from build123d import *

# Parameters (mm, degrees)
F1_DEPTH    = 19.05
F2_T2_ANGLE = 47.80727079
F4_DEPTH    = 3.175


# Not quite as in the source:
# - a fillet or chamfer that OpenCascade refuses, or shapes differently, is made with other operations: its cross-section is extruded or revolved along the edge and cut away or added


with BuildPart() as f1:
    # F0 (on Front) → F1 (new body)
    with BuildSketch(Plane.XZ):
        with BuildLine():
            Line((-379.386894745, -118.26875), (379.4125, -118.26875))
            Line((379.4125, -118.26875), (379.4125, -113.50625))
            Line((379.4125, -113.50625), (393.7, -113.50625))
            Line((393.7, -113.50625), (393.7, 124.61875))
            ThreePointArc((393.7, 124.61875), (-0.5889314831, 196.0563533265), (-393.674394745, 118.26875))
            Line((-393.674394745, 118.26875), (-393.674394745, -113.50625))
            Line((-393.674394745, -113.50625), (-379.386894745, -113.50625))
            Line((-379.386894745, -113.50625), (-379.386894745, -118.26875))
        make_face()
        with BuildLine():
            ThreePointArc((-393.674394745, 118.26875), (-0.5889314831, 196.0563533265), (393.7, 124.61875))
            Line((393.7, 124.61875), (393.7, 138.90625))
            ThreePointArc((393.7, 138.90625), (-0.7824585401, 208.7544433839), (-393.7768174305, 130.96875))
            Line((-393.7768174305, 130.96875), (-393.674394745, 118.26875))
        make_face()
    extrude(amount=F1_DEPTH)

    # F2: chamfer of 19.558 x 11.43 on 1 edges, made by hand

    # F2_s1 → F2_t2 (revolve, cut)
    with BuildSketch(Plane(origin=(327.911656241, 0, -141.3984070605), x_dir=(0, 1, 0), z_dir=(0.9182658757, 0, -0.3959643691))):
        Polygon((0.508, 284.621375818), (-19.05, 273.191375818), (-19.05, 284.621375818), align=None)
    revolve(axis=Axis((10.1741912427, -19.05, -878.2512511865), (0, -1, 0)), revolution_arc=F2_T2_ANGLE, mode=Mode.SUBTRACT)

    # F3 (on face) → F4 (join)
    with BuildSketch(Plane.XZ.offset(19.05)):
        Polygon((71.1841804533, -118.26875), (178.9472539061, -118.26875), (218.205169263, -79.0108346431), (164.3236325366, -25.1292979167), (110.4420958102, -79.0108346431), align=None)
        Polygon((218.205169263, -79.0108346431), (178.9472539061, -118.26875), (257.4630846199, -118.26875), align=None)
        Polygon((393.7, -113.50625), (393.7, -38.9795184745), (379.8497794422, -25.1292979167), (325.9682427158, -79.0108346431), (286.710327359, -118.26875), (379.4125, -118.26875), (379.4125, -113.50625), align=None)
        Polygon((379.8497794422, -25.1292979167), (393.7, -38.9795184745), (393.7, -11.279077359), align=None)
        Polygon((218.205169263, -79.0108346431), (257.4630846199, -118.26875), (286.710327359, -118.26875), (325.9682427158, -79.0108346431), (272.0867059894, -25.1292979167), (218.205169263, 28.7522388097), (164.3236325366, -25.1292979167), align=None)
        Polygon((41.9369377142, -118.26875), (71.1841804533, -118.26875), (110.4420958102, -79.0108346431), (56.5605590837, -25.1292979167), (2.6790223573, 28.7522388097), (-51.2025143691, -25.1292979167), (2.6790223573, -79.0108346431), align=None)
        Polygon((-36.5788929995, -118.26875), (41.9369377142, -118.26875), (2.6790223573, -79.0108346431), align=None)
        Polygon((-144.3419664524, -118.26875), (-36.5788929995, -118.26875), (2.6790223573, -79.0108346431), (-51.2025143691, -25.1292979167), (-105.0840510955, -79.0108346431), align=None)
        Polygon((325.9682427158, -79.0108346431), (379.8497794422, -25.1292979167), (393.7, -11.279077359), (393.7, 68.7835549784), (379.8497794422, 82.6337755361), (325.9682427158, 28.7522388097), (272.0867059894, -25.1292979167), align=None)
        Polygon((110.4420958102, -79.0108346431), (164.3236325366, -25.1292979167), (218.205169263, 28.7522388097), (164.3236325366, 82.6337755361), (110.4420958102, 28.7522388097), (56.5605590837, -25.1292979167), align=None)
        Polygon((-173.5892091915, -118.26875), (-144.3419664524, -118.26875), (-105.0840510955, -79.0108346431), (-158.9655878219, -25.1292979167), (-212.8471245483, 28.7522388097), (-266.7286612747, -25.1292979167), (-212.8471245483, -79.0108346431), align=None)
        Polygon((379.8497794422, 82.6337755361), (393.7, 68.7835549784), (393.7, 96.4839960939), align=None)
        Polygon((218.205169263, 28.7522388097), (272.0867059894, -25.1292979167), (325.9682427158, 28.7522388097), (272.0867059894, 82.6337755361), (218.205169263, 136.5153122625), (164.3236325366, 82.6337755361), align=None)
        Polygon((2.6790223573, 28.7522388097), (56.5605590837, -25.1292979167), (110.4420958102, 28.7522388097), (56.5605590837, 82.6337755361), (2.6790223573, 136.5153122625), (-51.2025143691, 82.6337755361), align=None)
        Polygon((-105.0840510955, -79.0108346431), (-51.2025143691, -25.1292979167), (2.6790223573, 28.7522388097), (-51.2025143691, 82.6337755361), (-105.0840510955, 28.7522388097), (-158.9655878219, -25.1292979167), align=None)
        Polygon((-252.1050399052, -118.26875), (-173.5892091915, -118.26875), (-212.8471245483, -79.0108346431), align=None)
        Polygon((-359.868113358, -118.26875), (-252.1050399052, -118.26875), (-212.8471245483, -79.0108346431), (-266.7286612747, -25.1292979167), (-320.6101980012, -79.0108346431), align=None)
        with BuildLine():
            Line((325.9682427158, 28.7522388097), (379.8497794422, 82.6337755361))
            Line((379.8497794422, 82.6337755361), (393.7, 96.4839960939))
            Line((393.7, 96.4839960939), (393.7, 126.6814901711))
            ThreePointArc((393.7, 126.6814901711), (365.104665334, 137.1335129285), (336.2249713921, 146.7720409389))
            Line((336.2249713921, 146.7720409388), (325.9682427158, 136.5153122625))
            Line((325.9682427158, 136.5153122625), (272.0867059894, 82.6337755361))
            Line((272.0867059894, 82.6337755361), (325.9682427158, 28.7522388097))
        make_face()
        with BuildLine():
            Line((110.4420958102, 28.7522388097), (164.3236325366, 82.6337755361))
            Line((164.3236325366, 82.6337755361), (218.205169263, 136.5153122625))
            Line((218.205169263, 136.5153122625), (169.1544903585, 185.565991167))
            ThreePointArc((169.1544903585, 185.565991167), (164.9380697375, 186.1875692954), (160.7192193307, 186.792435783))
            Line((160.7192193307, 186.792435783), (110.4420958102, 136.5153122625))
            Line((110.4420958102, 136.5153122625), (56.5605590837, 82.6337755361))
            Line((56.5605590837, 82.6337755361), (110.4420958102, 28.7522388097))
        make_face()
        Polygon((-212.8471245483, 28.7522388097), (-158.9655878219, -25.1292979167), (-105.0840510955, 28.7522388097), (-158.9655878219, 82.6337755361), (-212.8471245483, 136.5153122625), (-266.7286612747, 82.6337755361), align=None)
        with BuildLine():
            Line((218.205169263, 136.5153122625), (272.0867059894, 82.6337755361))
            Line((272.0867059894, 82.6337755361), (325.9682427158, 136.5153122625))
            Line((325.9682427158, 136.5153122625), (306.8177631195, 155.6657918589))
            ThreePointArc((306.8177631195, 155.6657918589), (238.4761479453, 172.8719942997), (169.1544903585, 185.565991167))
            Line((169.1544903585, 185.565991167), (218.205169263, 136.5153122625))
        make_face()
        with BuildLine():
            Line((2.6790223573, 136.5153122625), (56.5605590838, 82.6337755361))
            Line((56.5605590837, 82.6337755361), (110.4420958102, 136.5153122625))
            Line((110.4420958102, 136.5153122625), (56.5605590837, 190.3968489889))
            Line((56.5605590837, 190.3968489889), (50.3274681554, 196.6299399173))
            ThreePointArc((50.3274681554, 196.6299399173), (2.3207372282, 197.350991232), (-45.670346508, 195.92901685))
            Line((-45.670346508, 195.92901685), (-51.2025143691, 190.3968489889))
            Line((-51.2025143691, 190.3968489889), (2.6790223573, 136.5153122625))
        make_face()
        Polygon((-105.0840510955, 28.7522388097), (-51.2025143691, 82.6337755361), (2.6790223573, 136.5153122625), (-51.2025143691, 190.3968489889), (-105.0840510955, 136.5153122625), (-158.9655878219, 82.6337755361), align=None)
        Polygon((-266.7286612747, -25.1292979167), (-212.8471245483, 28.7522388097), (-266.7286612747, 82.6337755361), (-320.6101980012, 28.7522388097), (-374.4917347276, -25.1292979167), (-320.6404889111, -78.9805437332), (-320.6101980012, -79.0108346431), align=None)
        Polygon((-379.386894745, -118.26875), (-359.9286951779, -118.26875), (-320.6404889111, -78.9805437332), (-374.4917347276, -25.1292979167), (-393.674394745, -5.9466378993), (-393.674394745, -113.50625), (-379.386894745, -113.50625), align=None)
        with BuildLine():
            Line((325.9682427158, 136.5153122625), (336.2249713921, 146.7720409388))
            ThreePointArc((336.2249713921, 146.7720409389), (321.5531223101, 151.3239145605), (306.8177631195, 155.6657918589))
            Line((306.8177631195, 155.6657918589), (325.9682427158, 136.5153122625))
        make_face()
        with BuildLine():
            Line((56.5605590837, 190.3968489889), (110.4420958102, 136.5153122625))
            Line((110.4420958102, 136.5153122625), (160.7192193307, 186.792435783))
            ThreePointArc((160.7192193307, 186.792435783), (111.6070850178, 192.5863782868), (62.2805468294, 196.1168367345))
            Line((62.2805468293, 196.1168367345), (56.5605590837, 190.3968489889))
        make_face()
        with BuildLine():
            Line((-320.6101980012, 28.7522388097), (-266.7286612747, 82.6337755361))
            Line((-266.7286612747, 82.6337755361), (-212.8471245483, 136.5153122625))
            Line((-212.8471245483, 136.5153122625), (-243.3958660177, 167.0640537319))
            ThreePointArc((-243.3958660177, 167.0640537319), (-275.7499582928, 158.6813605815), (-307.8279930641, 149.2975171996))
            Line((-307.8279930641, 149.2975171996), (-320.6101980012, 136.5153122625))
            Line((-320.6101980012, 136.5153122625), (-374.4917347276, 82.6337755361))
            Line((-374.4917347276, 82.6337755361), (-320.6101980012, 28.7522388097))
        make_face()
        with BuildLine():
            Line((-212.8471245483, 136.5153122625), (-158.9655878219, 82.6337755361))
            Line((-158.9655878219, 82.6337755361), (-105.0840510955, 136.5153122625))
            Line((-105.0840510955, 136.5153122625), (-153.4329816595, 184.8642428265))
            ThreePointArc((-153.4329816595, 184.8642428265), (-198.6042128715, 176.9233498209), (-243.3958660177, 167.0640537319))
            Line((-243.3958660177, 167.0640537319), (-212.8471245483, 136.5153122625))
        make_face()
        with BuildLine():
            Line((50.3274681554, 196.6299399173), (56.5605590837, 190.3968489889))
            Line((56.5605590837, 190.3968489889), (62.2805468293, 196.1168367345))
            ThreePointArc((62.2805468294, 196.1168367345), (56.3047208944, 196.3900074992), (50.3274681554, 196.6299399173))
        make_face()
        with BuildLine():
            Line((-105.0840510955, 136.5153122625), (-51.2025143691, 190.3968489889))
            Line((-51.2025143691, 190.3968489889), (-45.670346508, 195.92901685))
            ThreePointArc((-45.670346508, 195.92901685), (-99.6910472687, 191.75411796), (-153.4329816595, 184.8642428265))
            Line((-153.4329816595, 184.8642428265), (-105.0840510955, 136.5153122625))
        make_face()
        Polygon((-374.4917347276, -25.1292979167), (-320.6101980012, 28.7522388097), (-374.4917347276, 82.6337755361), (-393.674394745, 101.8164355535), (-393.674394745, -5.9466378993), align=None)
        with BuildLine():
            Line((-393.674394745, 101.8164355535), (-374.4917347276, 82.6337755361))
            Line((-374.4917347276, 82.6337755361), (-320.6101980012, 136.5153122625))
            Line((-320.6101980012, 136.5153122625), (-327.1969421676, 143.102056429))
            ThreePointArc((-327.1969421676, 143.102056429), (-360.6383542509, 131.4417302391), (-393.6777661416, 118.6867895926))
            Line((-393.6777661416, 118.6867895926), (-393.674394745, 118.26875))
            Line((-393.674394745, 118.26875), (-393.674394745, 101.8164355535))
        make_face()
        with BuildLine():
            Line((-320.6101980012, 136.5153122625), (-307.8279930641, 149.2975171996))
            ThreePointArc((-307.8279930641, 149.2975171996), (-317.5271092238, 146.2455610624), (-327.1969421676, 143.102056429))
            Line((-327.1969421676, 143.102056429), (-320.6101980012, 136.5153122625))
        make_face()
    extrude(amount=F4_DEPTH)


solid = f1.part
For this review, take the finished solid that the model builds, in its own axes (mm). A direction names the side the tool comes from. Give positions to 0.01 mm unless a question says otherwise; leave off trailing zeros. Loops run counter-clockwise (first coordinate to the right, second up) from the corner with the lowest first, then second, coordinate; pieces in that order, holes last. Notation, with made-up numbers: (1.5, 58.5) - (24.5, 58.5) arc R19 ccw to (24.5, 77.5) - close; hole circle Ø11 at (23.5, -7.75). An arc over 180 degrees is marked (long way). Write each question's results on one line, items separated by ' | '.
(1) For faces 1 (the flat face through (386, -11, -113.506)), 2 (the flat face through (-387, -11, -113.506)), 3 (the flat face through (393.7, -11, 11)), list the 3-axis set-ups (+Z, -Z, +X, -X, +Y, -Y) from which the entire face can be reached by the end or side of a thin tool; tool diameter is ignored.
Conclusion:
face 1: -Z, +X, +Y, -Y | face 2: -Z, -X, +Y, -Y | face 3: +Z, -Z, +X, +Y, -Y
(2) For line 1 along X through (y, z) = (-10.75, 46); line 2 along Z through (x, y) = (134.5, -9.25); line 3 along Z through (x, y) = (-233, -6.25), list the stretches that pass through material, from the lowest coordinate up.
Conclusion:
line 1: -393.67 to 393.7 | line 2: -118.27 to 195.94 | line 3: -118.27 to 177.21
(3) For pin 1 Ø2 at (x, y) = (-13.5, -5.5) entering from +Z; pin 2 Ø7 at (x, y) = (-388.5, -16.5) entering from -Z; pin 3 Ø5 at (y, z) = (-6, 47.5) entering from -X, all flat-tipped, find the tip position at first contact; note any pin that passes through.
Conclusion:
pin 1: z = 205.62 | pin 2: z = -113.51 | pin 3: x = -393.67
(4) Take a section at A-A (y = -5.5). Give the boundary of the cut face in (x, z), then the cut area to 3 significant figures.
Conclusion:
outline: (-393.75, 127.2) - (-393.67, 118.27) - (-393.67, -113.51) - (-379.39, -113.51) - (-379.39, -118.27) - (379.41, -118.27) - (379.41, -113.51) - (393.7, -113.51) - (393.7, 135.15) arc R1083.55 ccw to start | area: 235,000 mm^2
